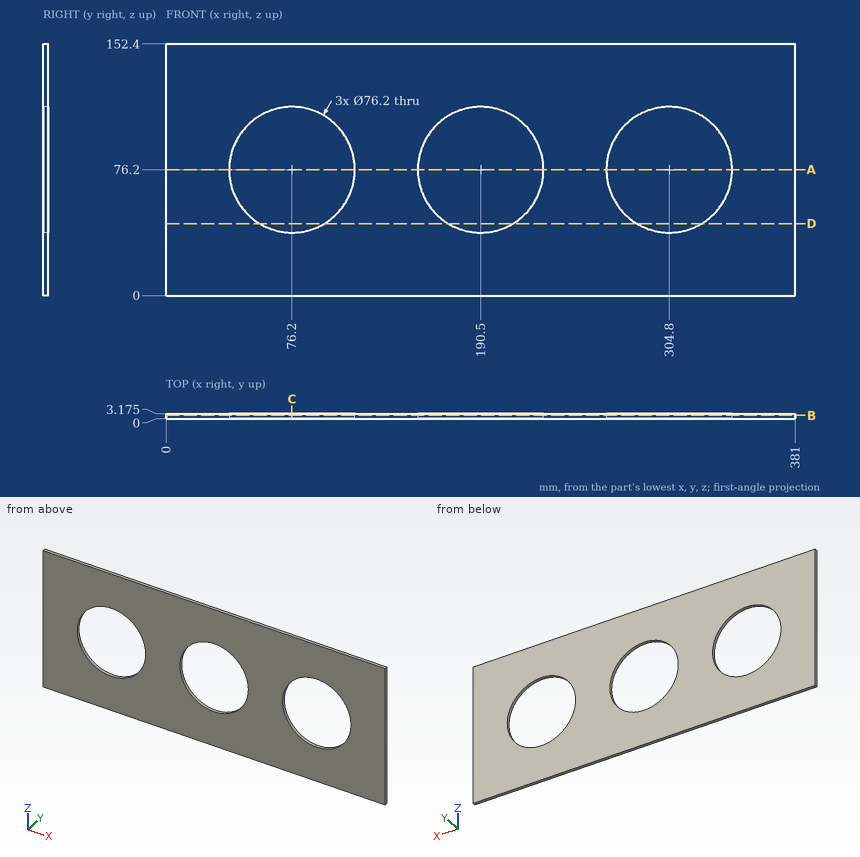
Job drawing, mm, ordinate dimensions from the low corner. One solid piece. Give positions to 0.01 mm unless a question says otherwise; leave off trailing zeros. Order: outer loops, then holes, each group sorted by start corner. A loop starts at its lowest first (then second) coordinate and runs counter-clockwise, first axis right, second up. Notation, with made-up numbers: M -1.5,89 L 42.5,89 A8 ccw 42.5,95 Z; hole C 3.5,82 d10. An arc over 180 degrees is marked long. Return JSON: item names as keys, results as strings.
Q1. Wall check: probe 1 along Z at (x, y) = (190.5, 1.2); probe 2 along X at (y, z) = (2.7, 83); probe 3 along Z at (x, y) = (328.5, 1.5). Give the ranges that are in metal, low to high. Write a range as from..to.
Answer list:
{"probe 1": "z = 0..38.1, 114.3..152.4", "probe 2": "x = 0..38.71, 113.69..153.01, 227.99..267.31, 342.29..381", "probe 3": "z = 0..46.37, 106.03..152.4"}
Q2. Band-saw the part on B-B (y = 2.05). Give the cut face in (x, z).
Answer list:
{"outline": "M 0,0 L 381,0 L 381,152.4 L 0,152.4 Z; hole C 76.2,76.2 d76.2; hole C 190.5,76.2 d76.2; hole C 304.8,76.2 d76.2"}
Q3. Band-saw the part on C-C (x = 76.2). Give the cut face in (y, z) (3 decimals), then the cut area to 3 significant figures.
Answer list:
{"outline": "M 0,0 L 3.175,0 L 3.175,38.1 L 0,38.1 Z; M 0,114.3 L 3.175,114.3 L 3.175,152.4 L 0,152.4 Z", "area": "242 mm^2"}
Q4. Band-saw the part on D-D (z = 43.5). Give the cut face in (x, y) (3 decimals).
Answer list:
{"outline": "M 0,0 L 56.647,0 L 56.647,3.175 L 0,3.175 Z; M 95.753,0 L 170.947,0 L 170.947,3.175 L 95.753,3.175 Z; M 210.053,0 L 285.247,0 L 285.247,3.175 L 210.053,3.175 Z; M 324.353,0 L 381,0 L 381,3.175 L 324.353,3.175 Z"}
Q5. Band-saw the part on A-A (z = 76.2). Give the cut face in (x, y) (3 decimals), then the cut area to 3 significant figures.
Answer list:
{"outline": "M 0,0 L 38.1,0 L 38.1,3.175 L 0,3.175 Z; M 114.3,0 L 152.4,0 L 152.4,3.175 L 114.3,3.175 Z; M 228.6,0 L 266.7,0 L 266.7,3.175 L 228.6,3.175 Z; M 342.9,0 L 381,0 L 381,3.175 L 342.9,3.175 Z", "area": "484 mm^2"}
